Here's how the part is built. I have some questions about the finished solid (model axes, mm). A direction names the side the tool comes from. Coordinates: 2 decimals unless noted, no trailing zeros. Write each loop counter-clockwise with the first axis right and the second up, starting at its lowest first coordinate (ties: lowest second). Pieces come first, ordered by that corner, then holes.
(1) Imagine slicing it at C-C, the plane z = 30. List the corners of the cut face in (x, y) for me, plus the area to 3 significant figures.
(2) For pin 1 Ø8 at (x, y) = (-35, -36.5) entering from +Z; pin 2 Ø11 at (x, z) = (-39.5, 28) entering from -Y; pin 3 Ø3 at (x, y) = (-22, -4) entering from -Z, each with a flat end and sliding along its axis, tell me the tip position at first contact or that it passes through.
(3) Please list where these lines run through material, in increasing order: probe 1 along Z at (x, y) = (-21.5, -36); probe 2 along Y at (x, z) = (-44, 4); probe 3 along Z at (x, y) = (-28.5, -32).
(4) Thinking about a two-plate mould opening in Y: for faces 1 (the flat face through (-43, 0, 20)), 2 (the flat face through (-20, -4, 34.08)), 3 (the flat face through (-12.373, -13.905, 20.409)), which applies, released by +Y, released by -Y, zero draft, split by the parting line, or undercut?
(5) Which directions (+Z, -Z, +X, -X, +Y, -Y) give clear straight access to the entire face, cutting with the end or side of a thin tool? Please do faces 4 (the cylindrical face through (-57.17, -44.76, 40.62)), 5 (the flat face through (-15, -39, 37)), 6 (the cylindrical face through (-56.302, -44.915, -0.625)).
(6) Imagine slicing it at D-D, the plane y = -23. List the corners of the cut face in (x, z) for me.
(7) Imagine slicing it at A-A, the plane y = -38. List the corners of the cut face in (x, z) for me.
```python
from build123d import *

# Parameters (mm, degrees)
SKETCH2_W                 = 70
SKETCH2_H                 = 35
BOSS_EXTRUDE2_DEPTH       = 40
SKETCH3_W                 = 28.105894453
SKETCH3_H                 = 27.971945797
CUT_EXTRUDE1_DEPTH        = 10
SKETCH4_R                 = 10
CUT_EXTRUDE2_DEPTH        = 3
CUT_EXTRUDE3_START        = -3
SKETCH5_R                 = 10
CUT_EXTRUDE3_DEPTH        = 3
BOSS_EXTRUDE3_DEPTH       = 3
BOSS_EXTRUDE3_DEPTH_BACK  = 3
SKETCH6_R                 = 10
SKETCH7_R                 = 10
BOSS_EXTRUDE5_DEPTH       = 6
SKETCH8_R                 = 2
CUT_EXTRUDE5_DEPTH        = 46
BOSS_EXTRUDE8_DEPTH       = 0.0001
BOSS_EXTRUDE8_DEPTH_BACK  = 46.0001
SKETCH9_R                 = 2
BOSS_EXTRUDE9_DEPTH       = 3
BOSS_EXTRUDE9_DEPTH_BACK  = 3
SKETCH10_R                = 10
BOSS_EXTRUDE10_DEPTH      = 3
BOSS_EXTRUDE10_DEPTH_BACK = 3
SKETCH11_R                = 10
SKETCH12_R                = 2
CUT_EXTRUDE6_DEPTH        = 46
BOSS_EXTRUDE11_DEPTH      = 0.001
BOSS_EXTRUDE11_DEPTH_BACK = 46.001
SKETCH13_R                = 2
BOSS_EXTRUDE12_DEPTH      = 28
SKETCH18_R                = 4
CUT_EXTRUDE11_DEPTH       = 10


with BuildPart() as part:
    # Sketch2 → Boss-Extrude2 (new body)
    with BuildSketch(Plane.XY):
        with Locations((-35, -17.5)):
            Rectangle(SKETCH2_W, SKETCH2_H)
    extrude(amount=BOSS_EXTRUDE2_DEPTH)

    # Sketch3 → Cut-Extrude1 (cut)
    with BuildSketch(Plane(origin=(0, 0, 0), x_dir=(1, 0, 0), z_dir=(0, 1, 0))):
        with Locations((-17.175677586, -20.094439992)):
            Rectangle(SKETCH3_W, SKETCH3_H)
    extrude(amount=-CUT_EXTRUDE1_DEPTH, mode=Mode.SUBTRACT)

    # Sketch4 → Cut-Extrude2 (cut)
    with BuildSketch(Plane.XY.offset(40)):
        with Locations((-15, -35)):
            Circle(SKETCH4_R)
        with Locations((-55, -35)):
            Circle(SKETCH4_R)
    extrude(amount=-CUT_EXTRUDE2_DEPTH, mode=Mode.SUBTRACT)

    # Sketch5 → Cut-Extrude3 (cut)
    with BuildSketch(Plane(origin=(0, 0, 0), x_dir=(-1, 0, 0), z_dir=(0, 0, -1)).offset(CUT_EXTRUDE3_START)):
        with Locations((15, -35)):
            Circle(SKETCH5_R)
        with Locations((55, -35)):
            Circle(SKETCH5_R)
    extrude(amount=CUT_EXTRUDE3_DEPTH, mode=Mode.SUBTRACT)

    # Sketch6 → Boss-Extrude3 (add, two sides: drawn at the far end of the back side and taken through both)
    with BuildSketch(Plane.XY.offset(40).offset(-BOSS_EXTRUDE3_DEPTH_BACK)):
        with Locations((-55, -35)):
            Circle(SKETCH6_R)
    extrude(amount=BOSS_EXTRUDE3_DEPTH + BOSS_EXTRUDE3_DEPTH_BACK)

    # Sketch7 → Boss-Extrude5 (add)
    with BuildSketch(Plane(origin=(0, 0, 3), x_dir=(-1, 0, 0), z_dir=(0, 0, -1))):
        with Locations(Location((55, -35, 0), (0, 0, 180))):
            Circle(SKETCH7_R)
    extrude(amount=BOSS_EXTRUDE5_DEPTH)

    # Sketch8 → Cut-Extrude5 (cut)
    with BuildSketch(Plane(origin=(0, 0, -3), x_dir=(-1, 0, 0), z_dir=(0, 0, -1))):
        with Locations((55, -35)):
            Circle(SKETCH8_R)
    extrude(amount=-CUT_EXTRUDE5_DEPTH, mode=Mode.SUBTRACT)

    # Sketch9 → Boss-Extrude8 (add, two sides: drawn at the far end of the back side and taken through both)
    with BuildSketch(Plane(origin=(0, 0, -3), x_dir=(-1, 0, 0), z_dir=(0, 0, -1)).offset(-BOSS_EXTRUDE8_DEPTH_BACK)):
        with Locations((55, -35)):
            Circle(SKETCH9_R)
    extrude(amount=BOSS_EXTRUDE8_DEPTH + BOSS_EXTRUDE8_DEPTH_BACK)

    # Sketch10 → Boss-Extrude9 (add, two sides: drawn at the far end of the back side and taken through both)
    with BuildSketch(Plane.XY.offset(40).offset(-BOSS_EXTRUDE9_DEPTH_BACK)):
        with Locations((-15, -35)):
            Circle(SKETCH10_R)
    extrude(amount=BOSS_EXTRUDE9_DEPTH + BOSS_EXTRUDE9_DEPTH_BACK)

    # Sketch11 → Boss-Extrude10 (add, two sides: drawn at the far end of the back side and taken through both)
    with BuildSketch(Plane(origin=(0, 0, 0), x_dir=(-1, 0, 0), z_dir=(0, 0, -1)).offset(-BOSS_EXTRUDE10_DEPTH_BACK)):
        with Locations(Location((15, -35, 0), (0, 0, 180))):
            Circle(SKETCH11_R)
    extrude(amount=BOSS_EXTRUDE10_DEPTH + BOSS_EXTRUDE10_DEPTH_BACK)

    # Sketch12 → Cut-Extrude6 (cut)
    with BuildSketch(Plane(origin=(0, 0, -3), x_dir=(-1, 0, 0), z_dir=(0, 0, -1))):
        with Locations((15, -35)):
            Circle(SKETCH12_R)
    extrude(amount=-CUT_EXTRUDE6_DEPTH, mode=Mode.SUBTRACT)

    # Sketch13 → Boss-Extrude11 (add, two sides: drawn at the far end of the back side and taken through both)
    with BuildSketch(Plane(origin=(0, 0, -3), x_dir=(-1, 0, 0), z_dir=(0, 0, -1)).offset(-BOSS_EXTRUDE11_DEPTH_BACK)):
        with Locations((15, -35)):
            Circle(SKETCH13_R)
    extrude(amount=BOSS_EXTRUDE11_DEPTH + BOSS_EXTRUDE11_DEPTH_BACK)

    # Sketch14 → Boss-Extrude12 (add)
    with BuildSketch(Plane(origin=(0, 0, 34.080412891), x_dir=(-1, 0, 0), z_dir=(0, 0, -1))):
        Polygon((3.122730359, 0), (31.228624812, -10), (3.122730359, -10), align=None)
    extrude(amount=BOSS_EXTRUDE12_DEPTH)

    # Sketch18 → Cut-Extrude11 (cut)
    with BuildSketch(Plane(origin=(-0.350891722, 0.986212569, 0), x_dir=(0.9421427910100845, 0.33521181564456864, 0), z_dir=(-0.33521181564456864, 0.9421427910100845, 0))):
        with Locations(Location((-16.374329601, -20.352535637, 0), (0, 0, 180))):
            Circle(SKETCH18_R)
    extrude(amount=-CUT_EXTRUDE11_DEPTH, mode=Mode.SUBTRACT)


solid = part.part
```
Recorded:
1. outline: (-70, -35) - (-57, -35) arc R2 ccw to (-53, -35) - (-17, -35) arc R2 ccw to (-13, -35) - (0, -35) - (0, 0) - (-3.12, 0) - (-31.23, -10) - (-31.23, 0) - (-70, 0) - close
1. area: 2,320 mm2
2. pin 1: stops at z = 40
2. pin 2: stops at y = -35
2. pin 3: stops at z = 0
3. probe 1: z = -3 to 3, 37 to 43
3. probe 2: y = -35 to 0
3. probe 3: z = 0 to 40
4. face 1: released by +Y
4. face 2: zero draft
4. face 3: undercut
5. face 4: +Z
5. face 5: -Y
5. face 6: -Z
6. outline: (-70, 0) - (0, 0) - (0, 40) - (-70, 40) - close
7. outline: (-64.54, -3) - (-45.46, -3) - (-45.46, 3) - (-64.54, 3) - close; (-64.54, 37) - (-45.46, 37) - (-45.46, 43) - (-64.54, 43) - close; (-24.54, -3) - (-5.46, -3) - (-5.46, 3) - (-24.54, 3) - close; (-24.54, 37) - (-5.46, 37) - (-5.46, 43) - (-24.54, 43) - close
